Can you work these out from the model? Positions are in its coordinate system, mm. A direction names the side the tool comes from. Round coordinates to 2 decimals unless told otherwise and drop trailing zeros. Order: outer loops, then holes, each group sorted by start corner. A loop starts at its lowest first (then second) coordinate and runs counter-clockwise, first axis right, second up. Notation, with made-up numbers: M -23,-29.5 L -17,-29.5 A29 ccw -17,3.5 Z; hole C 24.5,-27 d2. An arc over 180 degrees is marked long. One line per question, with ' | ' between items.
Autodesk Inventor part; units mm, degrees
ref_plane "YZ Plane" through (0, 0, 0) normal (1, 0, 0) x (0, 1, 0)
ref_plane "XZ Plane" through (0, 0, 0) normal (0, 1, 0) x (-1, 0, 0)
ref_plane "XY Plane" through (0, 0, 0) normal (0, 0, 1) x (1, 0, 0)
sketch "Эскиз2" plane through (0, 0, 0) normal (0, 0, 1) x (1, 0, 0)
  line L0 (-4.5, 3.25) -> (4.5, 3.25)
  line L1 (4.5, 3.25) -> (4.5, -3.25)
  line L2 (4.5, -3.25) -> (-4.5, -3.25)
  line L3 (-4.5, -3.25) -> (-4.5, 3.25)
  line L4 (-4.5, 3.25) -> (4.5, -3.25) construction
  line L5 (4.5, 3.25) -> (-4.5, -3.25) construction
  line L6 (8.5, 9.25) -> (4.5, 9.25) construction
  line L7 (-8.5, 9.25) -> (-8.5, -5.25)
  line L8 (-8.5, -5.25) -> (4.5, -5.25)
  line L9 (8.5, -5.25) -> (8.5, 9.25) construction
  line L10 (4.5, 3.25) -> (4.5, 9.25)
  line L11 (4.5, -3.25) -> (4.5, -5.25)
  line L12 (4.5, 9.25) -> (-8.5, 9.25)
  line L13 (4.5, -5.25) -> (8.5, -5.25) construction
  point P0 (0, 0)
  dimension "d0" = 9
  dimension "d1" = 6.5
  dimension "d2" = 6
extrude "Выдавливание1" add sketch "Эскиз2" along normal blind 14 contours L3 L2 L11 L8 L7 L12 L10 L0
sketch "Эскиз3" plane through (-8.5, 9.25, 0) normal (0, 1, 0) x (1, 0, 0)
  line L0 (13, 0) -> (0, 0) construction
  circle A0 centre (8.695, -6.5) radius 1.75
  line L1 (13, 0) -> (13, -14)
  point P0 (8.5, 0)
  dimension "d5" = 3.5
  dimension "d9" = 4.305
extrude "Выдавливание2" cut sketch "Эскиз3" against normal blind 20
sketch "Эскиз4" plane through (0, 0, 0) normal (0, 0, -1) x (-1, 0, 0)
  line L0 (2.9551, -1.2625) -> (2.9551, -1.7625) construction
  line L1 (2.9551, -1.7625) -> (3.4551, -1.7625) construction
  arc A0 (3.4551, -1.7625) -> (4.305, -2.445) centre (4.405, -1.45) ccw construction
  line L2 (4.305, -2.445) -> (4.305, -3.05) construction
  line L3 (4.305, -3.05) -> (4.105, -3.25) construction
  line L4 (4.105, -3.25) -> (-4.495, -3.25) construction
  line L5 (-4.495, -3.25) -> (-4.695, -3.05) construction
  line L6 (-4.695, -3.05) -> (-4.695, -2.445) construction
  arc A1 (-4.695, -2.445) -> (-3.8451, -1.7625) centre (-4.795, -1.45) ccw construction
  line L7 (-3.8451, -1.7625) -> (-3.3451, -1.7625) construction
  line L8 (-3.3451, -1.7625) -> (-3.3451, -1.2625) construction
  line L9 (-3.3451, -1.2625) -> (-3.8127, -1.2625) construction
  arc A2 (-3.8127, -1.2625) -> (-4.695, -0.455) centre (-4.795, -1.45) ccw construction
  line L10 (-4.695, -0.455) -> (-4.695, 3.05) construction
  line L11 (-4.695, 3.05) -> (-4.495, 3.25) construction
  line L12 (-4.495, 3.25) -> (4.105, 3.25) construction
  line L13 (4.105, 3.25) -> (4.305, 3.05) construction
  line L14 (4.305, 3.05) -> (4.305, -0.455) construction
  arc A3 (4.305, -0.455) -> (3.4227, -1.2625) centre (4.405, -1.45) ccw construction
  line L15 (3.4227, -1.2625) -> (2.9551, -1.2625) construction
  line L16 (4.1878, 3.45) -> (-4.5778, 3.45) construction
  line L17 (-4.5778, 3.45) -> (-4.895, 3.1328) construction
  line L18 (-4.895, 3.1328) -> (-4.895, -0.6563) construction
  arc A4 (-3.9951, -1.4625) -> (-4.895, -0.6563) centre (-4.795, -1.45) ccw construction
  line L19 (-3.9951, -1.4625) -> (-3.5451, -1.4625) construction
  line L20 (-3.5451, -1.4625) -> (-3.5451, -1.5625) construction
  line L21 (-3.5451, -1.5625) -> (-4.0029, -1.5625) construction
  arc A5 (-4.895, -2.2437) -> (-4.0029, -1.5625) centre (-4.795, -1.45) ccw construction
  line L22 (-4.895, -2.2437) -> (-4.895, -3.1328) construction
  line L23 (-4.895, -3.1328) -> (-4.5778, -3.45) construction
  line L24 (-4.5, -3.45) -> (4.1878, -3.45)
  line L25 (4.1878, -3.45) -> (4.505, -3.1328)
  line L26 (4.505, -3.1328) -> (4.505, -2.2437)
  arc A6 (3.6129, -1.5625) -> (4.505, -2.2437) centre (4.405, -1.45) ccw
  line L27 (3.6129, -1.5625) -> (3.1551, -1.5625)
  line L28 (3.1551, -1.5625) -> (3.1551, -1.4625)
  line L29 (3.1551, -1.4625) -> (3.6051, -1.4625)
  arc A7 (4.505, -0.6563) -> (3.6051, -1.4625) centre (4.405, -1.45) ccw
  line L30 (4.505, -0.6563) -> (4.505, 3.1328)
  line L31 (4.505, 3.1328) -> (4.1878, 3.45)
  line L32 (4.1878, 3.45) -> (8.5, 3.45)
  line L33 (8.5, 9.25) -> (8.5, -5.25)
  line L34 (-4.5, -5.25) -> (-4.5, -3.25)
  line L35 (-4.5, -3.45) -> (-4.5, -29.05)
  line L36 (-4.5, -29.05) -> (10.5, -29.05)
  line L37 (10.5, -29.05) -> (10.5, 3.45)
  line L38 (10.5, 3.45) -> (8.5, 3.45)
  point P0 (0, 0)
  dimension "d10" = 0.2
  dimension "d12" = 4.3122
  dimension "d13" = 15
extrude "Выдавливание3" add sketch "Эскиз4" along normal blind 12.4 and the other way blind 3
chamfer "Фаска1" distance 2 angle 45 1 edges at (-8.5, 3.45, 1.5)
chamfer "Фаска2" distance 2 angle 45 1 edges at (-6.3439, 3.45, 0)
chamfer "Фаска3" distance 2 angle 45 1 edges at (-8.5, -0.9, 3)
ref_plane "РабПлоскость1" through (0, 0, -4.7) normal (0, 0, -1) x (-1, 0, 0)
sketch "Эскиз5" plane through (0, 0, -4.7) normal (0, 0, -1) x (-1, 0, 0)
  circle A0 centre (2.8764, -21.05) radius 11 construction
  line L0 (-4.5, -29.05) -> (10.5, -29.05) construction
  circle A1 centre (2.8764, -21.05) radius 1.6
  line L1 (10.5, -29.05) -> (10.5, 3.45)
  line L2 (10.5, -29.05) -> (10.5, -9.05)
  line L3 (10.5, -9.05) -> (-4.5, -9.05)
  line L4 (-4.5, -3.45) -> (-4.5, -29.05)
  line L5 (-4.5, -9.05) -> (-4.5, -29.05)
  line L6 (-4.5, -29.05) -> (10.5, -29.05)
  point P0 (0, 0)
  dimension "d27" = 22
  dimension "d28" = 8
  dimension "d29" = 3.2
  dimension "d30" = 12
extrude "Выдавливание4" cut sketch "Эскиз5" along normal mid plane 7.4
extrude "Выдавливание5" cut sketch "Эскиз5" along normal mid plane 20 contours A1
sketch "Эскиз6" plane through (0, 0, -12.4) normal (0, 0, -1) x (-1, 0, 0)
  circle A0 centre (2.8764, -21.05) radius 1.6 construction
  circle A1 centre (2.8764, -21.05) radius 1.6
  line L0 (4.5507, -23.95) -> (1.2021, -23.95)
  line L1 (1.2021, -23.95) -> (-0.4722, -21.05)
  line L2 (-0.4722, -21.05) -> (1.2021, -18.15)
  line L3 (1.2021, -18.15) -> (4.5507, -18.15)
  line L4 (4.5507, -18.15) -> (6.2251, -21.05)
  line L5 (6.2251, -21.05) -> (4.5507, -23.95)
  line L6 (-4.5, -29.05) -> (10.5, -29.05)
  point P0 (0, 0)
  dimension "d35" = 5.8
extrude "Выдавливание6" cut sketch "Эскиз6" against normal blind 2.4
chamfer "Фаска4" distance 2 angle 45 5 edges at (-10.5, -29.05, -10.4) (-10.5, -29.05, 1) (4.5, -29.05, 1) (4.5, -29.05, -10.4) (-7.3439, 3.45, -12.4)
properties part number "ограничитель" material "Полипропилен"
(1) If we section it at B-B on x = 0: Please give me the cut outline in (y, z).
Final values:
outline: M -29.05,-12.4 L -21.87,-12.4 L -21.87,-10 L -20.23,-10 L -20.23,-12.4 L -3.45,-12.4 L -3.45,0 L -3.25,0 L -3.25,4.76 L -5.25,4.76 L -5.25,3 L -29.05,3 L -29.05,-1 L -9.05,-1 L -9.05,-8.4 L -29.05,-8.4 Z; M -5.25,8.24 L -3.25,8.24 L -3.25,14 L -5.25,14 Z; M 3.25,0 L 9.25,0 L 9.25,4.76 L 3.25,4.76 Z; M 3.25,8.24 L 9.25,8.24 L 9.25,14 L 3.25,14 Z
(2) On a 3-axis mill with a long thin cutter (end or side, diameter ignored), from which of +Z, -Z, +X, -X, +Y, -Y can I reach the whole of each face in a straight line? I mean faces 1 (the cylindrical face through (-0.18, -4.24, 8.21)), 2 (the flat face through (-5.376, -19.58, -11.217)). Say none if no direction works.
Final values:
face 1: +Y, -Y | face 2: -Z
(3) Will these pins go through, and if not, where does the flat tip stop? pin 1 Ø1.5 at (x, y) = (-4, -11.5) entering from +Z; pin 2 Ø7 at (x, z) = (1, -9) entering from +Y; pin 3 Ø3 at (y, z) = (1.5, 4.5) entering from +X.
Final values:
pin 1: z = 3 | pin 2: y = -3.45 | pin 3: x = -4.5
(4) Please list where these lines run through material, in increasing order: probe 1 along Y at (x, z) = (-2.25, -10.5); probe 2 along Z at (x, y) = (0.75, -12); probe 3 along Y at (x, z) = (-1.25, 3.5). Write a range as [from, to].
Final values:
probe 1: [-29.05, -23.95], [-18.15, -3.45] | probe 2: [-12.4, -8.4], [-1, 3] | probe 3: [-5.25, -3.25], [3.25, 9.25]
(5) If we section it at C-C on y = -10: Please give me the cut outline in (x, z).
Final values:
outline: M -10.5,-12.4 L 4.5,-12.4 L 4.5,-8.4 L -10.5,-8.4 Z; M -10.5,-1 L 4.5,-1 L 4.5,3 L -10.5,3 Z
(6) If we section it at A-A on z = 6.5: Please give me the cut outline in (x, y) (3 decimals), plus the area to 3 significant figures.
Final values:
outline: M -8.5,-5.25 L -1.555,-5.25 L -1.555,-3.25 L -4.5,-3.25 L -4.5,3.25 L -1.555,3.25 L -1.555,9.25 L -8.5,9.25 Z; M 1.945,-5.25 L 4.5,-5.25 L 4.5,-3.25 L 1.945,-3.25 Z; M 1.945,3.25 L 4.5,3.25 L 4.5,9.25 L 1.945,9.25 Z | area: 102 mm^2
(7) If we section it at D-D on y = -20: Please give me the cut outline in (x, z).
Final values:
outline: M -10.5,-12.4 L -5.62,-12.4 L -5.62,-10 L -4.08,-10 L -4.08,-8.4 L -10.5,-8.4 Z; M -10.5,-1 L -4.08,-1 L -4.08,3 L -10.5,3 Z; M -1.67,-10 L -0.13,-10 L -0.13,-12.4 L 4.5,-12.4 L 4.5,-8.4 L -1.67,-8.4 Z; M -1.67,-1 L 4.5,-1 L 4.5,3 L -1.67,3 Z
(8) Thinking about a two-plate mould opening in Y: for faces 3 (the flat face through (-3, -16, 3)), 4 (the flat face through (-4.505, -2.7, -6.1)), 5 (the flat face through (-3, -5.25, 8)), which applies, released by +Y, released by -Y, zero draft, split by the parting line, or undercut?
Final values:
face 3: zero draft | face 4: undercut | face 5: released by -Y
